The listing builds one solid part. Answer for the finished solid, in the listing's coordinates (mm). Face numbers are marked on the shaded views. Give positions to 0.01 mm unless a question says otherwise; leave off trailing zeros. Write each loop counter-clockwise with the first axis right and the second up, starting at its lowest first coordinate (ties: lowest second). Pieces come first, ordered by that corner, then holes. Notation, with made-up numbers: (-33.5, 84.5) -> (-8.5, 84.5) arc R25 cw to (-8.5, 105.5) -> close; hole circle Ø1 at (83, 4). An arc over 180 degrees is marked (long way). Put each result on its own line as item: value. Start each with the question number.
1) A cutting plane is placed at B-B (x = -13.5). Write down the section's boundary in (y, z), then the cut area to 3 significant figures.
2) A cutting plane is placed at C-C (z = 2.5). Write down the section's boundary in (x, y).
3) A cutting plane is placed at D-D (y = -11.75). Write down the section's boundary in (x, z).
4) For a pull along Z with two mould halves and no side action, classify the marked faces 1, 2, 3 and 4 as released by +Z, released by -Z, zero draft, split by the parting line, or undercut.
5) Find the intervals of material crossed by line 1 along Z through (x, y) = (13.5, -1.5); line 2 along X through (y, z) = (0.25, 5); line 3 along Z through (x, y) = (-13.5, -3), in increasing order. Write a range as from..to.
6) A flat-ended cylindrical pin translates along its axis: pin 1 Ø2.5 at (x, z) = (13.5, 3.5) entering from +Y. Find the tip coordinate at first contact, or state that the pin passes through.
7) A cutting plane is placed at A-A (y = 0). Write down the section's boundary in (x, z).
from build123d import *

# Parameters (mm, degrees)
SKETCH_W        = 36
SKETCH_H        = 29
SKETCH_R        = 11
PAD_DEPTH       = 7
SKETCH001_R     = 2.1
SKETCH001_R_2   = 2.5
POCKET_DEPTH    = 29.001
CHAMFER_SIZE    = 1
CHAMFER001_SIZE = 1
CHAMFER002_SIZE = 1


with BuildPart() as part:
    # Sketch → Pad (new body)
    with BuildSketch(Plane.XY):
        Rectangle(SKETCH_W, SKETCH_H)
        Circle(SKETCH_R, mode=Mode.SUBTRACT)
    extrude(amount=PAD_DEPTH)

    # Sketch001 (on Face3 of Pad) → Pocket (cut, through all)
    with BuildSketch(Plane.XZ.offset(14.5)):
        with Locations((13.5, 3.5)):
            Circle(SKETCH001_R)
        with Locations((-13.5, 3.5)):
            Circle(SKETCH001_R_2)
    extrude(amount=-POCKET_DEPTH, mode=Mode.SUBTRACT)

    # Chamfer
    chamfer_edges = [part.edges().sort_by_distance(p)[0] for p in [
        (18, -14.5, 3.5),
    ]]
    chamfer(chamfer_edges, length=CHAMFER_SIZE)

    # Chamfer001
    chamfer001_edges = [part.edges().sort_by_distance(p)[0] for p in [
        (-18, -14.5, 3.5),
    ]]
    chamfer(chamfer001_edges, length=CHAMFER001_SIZE)

    # Chamfer002
    chamfer002_edges = [part.edges().sort_by_distance(p)[0] for p in [
        (18, 14.5, 3.5),
        (-18, 14.5, 3.5),
    ]]
    chamfer(chamfer002_edges, length=CHAMFER002_SIZE)


solid = part.part
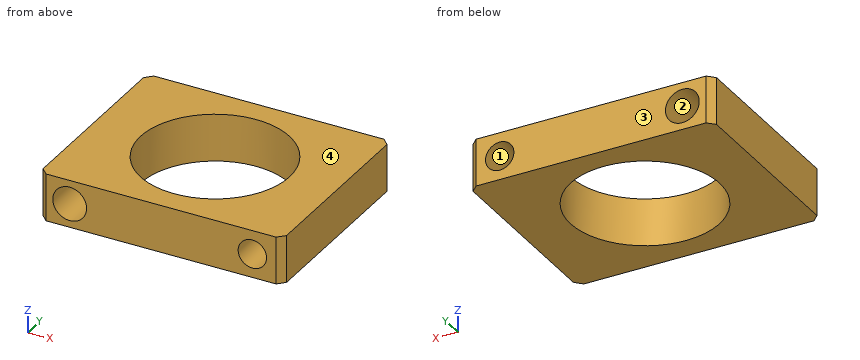
Reply:
1. outline: (-14.5, 0) -> (14.5, 0) -> (14.5, 1) -> (-14.5, 1) -> close; (-14.5, 6) -> (14.5, 6) -> (14.5, 7) -> (-14.5, 7) -> close
1. area: 58.0 mm2
2. outline: (-18, -13.5) -> (-17, -14.5) -> (-15.79, -14.5) -> (-15.79, 14.5) -> (-17, 14.5) -> (-18, 13.5) -> close; (-11.21, -14.5) -> (11.65, -14.5) -> (11.65, 14.5) -> (-11.21, 14.5) -> close; (15.35, -14.5) -> (17, -14.5) -> (18, -13.5) -> (18, 13.5) -> (17, 14.5) -> (15.35, 14.5) -> close; hole circle Ø22 at (0, 0)
3. outline: (-18, 0) -> (18, 0) -> (18, 7) -> (-18, 7) -> close; hole circle Ø5 at (-13.5, 3.5); hole circle Ø4.2 at (13.5, 3.5)
4. face 1: undercut
4. face 2: undercut
4. face 3: zero draft
4. face 4: released by +Z
5. line 1: z = 0..1.4, 5.6..7
5. line 2: x = -18..-15.5, -11.5..-11, 11..12.03, 14.97..18
5. line 3: z = 0..1, 6..7
6. pin 1: passes through
7. outline: (-18, 0) -> (-11, 0) -> (-11, 7) -> (-18, 7) -> close; (11, 0) -> (18, 0) -> (18, 7) -> (11, 7) -> close; hole circle Ø5 at (-13.5, 3.5); hole circle Ø4.2 at (13.5, 3.5)
